```python
from build123d import *

# Parameters (mm, degrees)
SKETCH1_R                = 1.5
SKETCH1_R_2              = 8.5
SKETCH1_W                = 6
SKETCH1_H                = 30
SKETCH1_W_2              = 22
SKETCH1_H_2              = 20
BOSS_EXTRUDE1_DEPTH      = 6
SKETCH1_5_W              = 6
SKETCH1_5_H              = 30
RESSALTO_EXTRUS_O1_DEPTH = 21.6
ESBO_O1_W                = 30
ESBO_O1_H                = 5
RESSALTO_EXTRUS_O2_DEPTH = 9
CORTE_EXTRUS_O1_REACH    = 79.561
ESBO_O2_W                = 5
ESBO_O2_H                = 15
FILETE2_R                = 2
FILETE2_OF_ESPELHAR1_R   = 2
FILLET1_R                = 3
FILETE1_R                = 2
ESBO_O4_W                = 2
ESBO_O4_H                = 4
ESBO_O4_W_2              = 45.13986754
CORTE_EXTRUS_O3_DEPTH    = 1.5
FILETE3_R                = 0.3


with BuildPart() as part:
    # Sketch1 → Boss-Extrude1 (new body)
    # profile 1 of 6: a face of its own
    with BuildSketch(Plane(origin=(0, 0, 0), x_dir=(1, 0, 0), z_dir=(0, 1, 0))):
        Polygon((-20.510374251, 47.623346162), (-8, 62), (8, 62), (20.489621783, 47.605313925), (20.489621783, 17.605313925), (11, 0), (-11, 0), (-20.510374251, 17.623346162), align=None)
        with Locations(Location((13.5, 37.605313925, 0), (0, 0, 270))):
            Circle(SKETCH1_R, mode=Mode.SUBTRACT)
        with Locations(Location((-13.5, 37.605313925, 0), (0, 0, 270))):
            Circle(SKETCH1_R, mode=Mode.SUBTRACT)
        with Locations(Location((5.25, 57.999859765, 0), (0, 0, 270))):
            Circle(SKETCH1_R, mode=Mode.SUBTRACT)
        with Locations(Location((-5.25, 57.999859765, 0), (0, 0, 270))):
            Circle(SKETCH1_R, mode=Mode.SUBTRACT)
        with Locations(Location((7.519679741, 17.780252273, 0), (0, 0, 270))):
            Circle(SKETCH1_R_2, mode=Mode.SUBTRACT)
        with Locations(Location((6, 4, 0), (0, 0, 270))):
            Circle(SKETCH1_R, mode=Mode.SUBTRACT)
        with Locations(Location((-6, 4, 0), (0, 0, 270))):
            Circle(SKETCH1_R, mode=Mode.SUBTRACT)
        with BuildLine():
            ThreePointArc((10.062695821, 30.018841621), (11.998189223, 31.105465162), (11.187975781, 33.171969363))
            ThreePointArc((11.187975781, 33.171969363), (9.667400631, 34.394210987), (8.730303993, 36.105313925))
            Line((8.730303993, 36.105313925), (-8.730303993, 36.105313925))
            ThreePointArc((-8.730303993, 36.105313925), (-10.541960108, 33.574185051), (-13.5, 32.605313925))
            Line((-13.5, 32.605313925), (-13.5, 17.787899155))
            ThreePointArc((-13.5, 17.787899155), (-9.241131059, 13.528058523), (-4.980318958, 17.785955551))
            ThreePointArc((-4.980318958, 17.785955551), (-0.366780245, 27.478383479), (10.062695821, 30.018841621))
        make_face(mode=Mode.SUBTRACT)
        with BuildLine():
            ThreePointArc((12.574074074, 42.518832133), (0, 51.105313925), (-12.574074074, 42.518832133))
            ThreePointArc((-12.574074074, 42.518832133), (-10.179901517, 41.34388933), (-8.730303993, 39.105313925))
            Line((-8.730303993, 39.105313925), (8.730303993, 39.105313925))
            ThreePointArc((8.730303993, 39.105313925), (10.179901517, 41.34388933), (12.574074074, 42.518832133))
        make_face(mode=Mode.SUBTRACT)
    # profile 2 of 6: a face of its own
    with BuildSketch(Plane(origin=(0, 0, 0), x_dir=(1, 0, 0), z_dir=(0, 1, 0))):
        Polygon((20.489621783, 17.605313925), (11, 0), (27.589621783, 0), (27.589621783, 30), (20.489621783, 30), align=None)
    # profile 3 of 6: a face of its own
    with BuildSketch(Plane(origin=(0, 0, 0), x_dir=(1, 0, 0), z_dir=(0, 1, 0))):
        with Locations((30.589621783, 15)):
            Rectangle(SKETCH1_W, SKETCH1_H)
    # profile 4 of 6: a face of its own
    with BuildSketch(Plane(origin=(0, 0, 0), x_dir=(1, 0, 0), z_dir=(0, 1, 0))):
        with Locations((0, -10)):
            Rectangle(SKETCH1_W_2, SKETCH1_H_2)
    # profile 5 of 6: a face of its own
    with BuildSketch(Plane(origin=(0, 0, 0), x_dir=(1, 0, 0), z_dir=(0, 1, 0))):
        Polygon((-31.550245757, 0), (-11, 0), (-20.510374251, 17.623346162), (-20.510374251, 30), (-31.550245757, 30), align=None)
    # profile 6 of 6: a face of its own
    with BuildSketch(Plane(origin=(0, 0, 0), x_dir=(1, 0, 0), z_dir=(0, 1, 0))):
        with Locations((-34.550245757, 15)):
            Rectangle(SKETCH1_W, SKETCH1_H)
    extrude(amount=BOSS_EXTRUDE1_DEPTH)

    # Sketch1<5> → Ressalto-extrusão1 (add)
    with BuildSketch(Plane(origin=(0, 0, 0), x_dir=(1, 0, 0), z_dir=(0, 1, 0))):
        with Locations((30.589621783, 15)):
            Rectangle(SKETCH1_5_W, SKETCH1_5_H)
    ressalto_extrus_o1 = extrude(amount=-RESSALTO_EXTRUS_O1_DEPTH)

    # Esboço1 → Ressalto-extrusão2 (add)
    with BuildSketch(Plane.ZY.offset(-27.589621783)):
        with Locations((-15, -19.1)):
            Rectangle(ESBO_O1_W, ESBO_O1_H)
    ressalto_extrus_o2 = extrude(amount=RESSALTO_EXTRUS_O2_DEPTH)

    # Esboço2 → Corte-extrusão1 (cut, up to next)
    with BuildSketch(Plane.XZ.offset(21.6), mode=Mode.PRIVATE) as corte_extrus_o1_sk1:
        with Locations((23.089621783, -17.9)):
            Rectangle(ESBO_O2_W, ESBO_O2_H)
    corte_extrus_o1_tool1 = extrude(corte_extrus_o1_sk1.sketch, amount=-CORTE_EXTRUS_O1_REACH, mode=Mode.PRIVATE) & part.part
    corte_extrus_o1 = corte_extrus_o1_tool1.solids().sort_by_distance((23.089622, -21.6, -17.9))[0]
    add(corte_extrus_o1, mode=Mode.SUBTRACT)

    # Filete2
    filete2_edges = [part.edges().sort_by_distance(p)[0] for p in [
        (25.589621783, -19.1, -25.4),
        (25.589621783, -19.1, -10.4),
        (20.589621783, -19.1, -10.4),
        (20.589621783, -19.1, -25.4),
    ]]
    fillet(filete2_edges, radius=FILETE2_R)

    # Espelhar1: Ressalto-extrusão1, Ressalto-extrusão2, Corte-extrusão1 across plane
    add(ressalto_extrus_o1.mirror(Plane.ZY.offset(1.980311987)))
    add(ressalto_extrus_o2.mirror(Plane.ZY.offset(1.980311987)))
    add(corte_extrus_o1.mirror(Plane.ZY.offset(1.980311987)), mode=Mode.SUBTRACT)

    # Filete2 of Espelhar1
    filete2_of_espelhar1_edges = [part.edges().sort_by_distance(p)[0] for p in [
        (-29.550245757, -19.1, -25.4),
        (-29.550245757, -19.1, -10.4),
        (-24.550245757, -19.1, -10.4),
        (-24.550245757, -19.1, -25.4),
    ]]
    fillet(filete2_of_espelhar1_edges, radius=FILETE2_OF_ESPELHAR1_R)

    # Fillet1
    fillet1_edges = [part.edges().sort_by_distance(p)[0] for p in [
        (-20.510374251, 3, -47.623346162),
        (-8, 3, -62),
        (8, 3, -62),
        (20.489621783, 3, -47.605313925),
        (20.489621783, 3, -30),
        (33.589621783, -7.8, -30),
        (33.589621783, -7.8, 0),
        (-37.550245757, -7.8, 0),
        (-37.550245757, -7.8, -30),
        (-20.510374251, 3, -30),
    ]]
    fillet(fillet1_edges, radius=FILLET1_R)

    # Filete1
    filete1_edges = [part.edges().sort_by_distance(p)[0] for p in [
        (27.589621783, 0, -15),
        (27.589621783, -16.6, -15),
        (-31.550245757, 0, -15),
        (-31.550245757, -16.6, -15),
    ]]
    fillet(filete1_edges, radius=FILETE1_R - 0.0001)  # a hair under: the kernel refuses the full size

    # Esboço4 → Corte-extrusão3 (cut)
    with BuildSketch(Plane.XZ.offset(21.6)):
        with Locations((-23.550245757, -17.9)):
            Rectangle(ESBO_O4_W, ESBO_O4_H)
        with Locations((0.019688013, -17.9)):
            Rectangle(ESBO_O4_W_2, ESBO_O4_H)
    extrude(amount=-CORTE_EXTRUS_O3_DEPTH, mode=Mode.SUBTRACT)

    # Filete3
    filete3_edges = [part.edges().sort_by_distance(p)[0] for p in [
        (19.589621783, -20.1, -19.9),
        (-23.550245757, -20.1, -19.9),
        (19.589621783, -20.1, -15.9),
        (-23.550245757, -20.1, -15.9),
    ]]
    fillet(filete3_edges, radius=FILETE3_R)


solid = part.part
```
Work out the finished part from the listing and answer in its coordinate system (mm). A direction names the side the tool comes from. Give positions to 0.01 mm unless a question says otherwise; leave off trailing zeros. Order: outer loops, then holes, each group sorted by start corner. A loop starts at its lowest first (then second) coordinate and runs counter-clockwise, first axis right, second up. Notation, with made-up numbers: (63.5, 40.25) -> (96.5, 40.25) arc R24 ccw to (96.5, 61.25) -> close; hole circle Ø10 at (-22.5, 15.5). An arc over 180 degrees is marked (long way). Answer as CSV lines item,"result". Start each with the question number.
(1) Consider line 1 along X through (y, z) = (1.25, -4); line 2 along Y through (x, z) = (19, -25); line 3 along X through (y, z) = (-12.5, -23). Determine where each line is inside the solid, lowest interval first.
(2) Section B-B, the plane z = -4 is taken. Write down the section's boundary in (x, y), plus the area to 3 significant figures.
(3) Section C-C, the plane x = 13.5 is taken. Write down the section's boundary in (y, z), plus the area to 3 significant figures.
(4) Section D-D, the plane z = -41 is taken. Write down the section's boundary in (x, y).
(5) For a pull along Y with two mould halves and no side action, classify faces 5 (the flat face through (-14.411, 2.958, -54.632)), 6 (the flat face through (20, -16.6, -15)), 7 (the flat face through (-30, -21.6, -15)) as released by +Y, released by -Y, zero draft, split by the parting line, or undercut.
(6) Each of these flat-tipped pins is pushed along its axis until it touches: pin 1 Ø6.5 at (y, z) = (2, -38.5) entering from -X; pin 2 Ø3.5 at (x, z) = (13.5, -37.61) entering from -Y; pin 3 Ø5 at (x, z) = (-6.5, -41.5) entering from +Y; pin 4 Ø0.8 at (x, y) = (-27, -20) entering from +Z. Where does it stop, or does it pass through?
(7) Section A-A, the plane y = -7 is taken. Write down the section's boundary in (x, z), plus the area to 3 significant figures.
(8) Which of the six approach directions +Z, -Z, +X, -X, +Y, -Y give full straight-line access (tool end or side, diameter ignored) to faces 1 (the flat face through (0, 3, -39.105)), 2 (the flat face through (29, -11, -30)), 3 (the cylindrical face through (21.16, -19.07, -24.8)), 4 (the flat face through (-20.51, 3, -40))?
Entries:
1,line 1,"-37.55 to -7.5, -4.5 to 4.5, 7.5 to 33.59"
1,line 2,"-21.6 to -16.6, 0 to 6"
1,line 3,"-37.55 to -31.55, 27.59 to 33.59"
2,outline,"(-37.55, -21.6) -> (-22.55, -21.6) -> (-22.55, -16.6) -> (-29.55, -16.6) arc R2 cw to (-31.55, -14.6) -> (-31.55, -2) arc R2 cw to (-29.55, 0) -> (-7.5, 0) -> (-7.5, 6) -> (-37.55, 6) -> close; (-4.5, 0) -> (4.5, 0) -> (4.5, 6) -> (-4.5, 6) -> close; (7.5, 0) -> (25.59, 0) arc R2 cw to (27.59, -2) -> (27.59, -14.6) arc R2 cw to (25.59, -16.6) -> (18.59, -16.6) -> (18.59, -21.6) -> (33.59, -21.6) -> (33.59, 6) -> (7.5, 6) -> close"
2,area,"743 mm²"
3,outline,"(0, -55.66) -> (6, -55.66) -> (6, -39.11) -> (0, -39.11) -> close; (0, -36.11) -> (6, -36.11) -> (6, -23.82) -> (0, -23.82) -> close; (0, -11.74) -> (6, -11.74) -> (6, 0) -> (0, 0) -> close"
3,area,"243 mm²"
4,outline,"(-20.51, 0) -> (-9.83, 0) -> (-9.83, 6) -> (-20.51, 6) -> close; (9.83, 0) -> (20.49, 0) -> (20.49, 6) -> (9.83, 6) -> close"
5,face 5,"zero draft"
5,face 6,"undercut"
5,face 7,"released by -Y"
6,pin 1,"x = -20.51"
6,pin 2,"y = 0"
6,pin 3,"y = 6"
6,pin 4,"z = 0"
7,outline,"(-37.55, -27) arc R3 ccw to (-34.55, -30) -> (-31.55, -30) -> (-31.55, 0) -> (-34.55, 0) arc R3 ccw to (-37.55, -3) -> close; (27.59, -30) -> (30.59, -30) arc R3 ccw to (33.59, -27) -> (33.59, -3) arc R3 ccw to (30.59, 0) -> (27.59, 0) -> close"
7,area,"352 mm²"
8,face 1,"+Y, -Y"
8,face 2,"-Z, +X, -Y"
8,face 3,"-Y"
8,face 4,"-Z, -X, +Y, -Y"
